```python
from build123d import *

# Parameters (mm, degrees)
F0_R     = 10.7663
F1_DEPTH = 30
F2_DEPTH = 60


# Not quite as in the source:
# - ends of sketch curves that miss each other by under 0.0002 mm in the source are joined


with BuildPart() as f1:
    # F0 (on Front) → F1 (new body)
    with BuildSketch(Plane.XZ):
        with BuildLine():
            ThreePointArc((3.5818546953, 22.2130663561), (17.1295319645, 14.5886645954), (22.5, 0))
            ThreePointArc((22.5, 0), (17.1295319492, -14.5886646134), (3.5818546487, -22.2130663636))
            Line((3.5818546487, -22.2130663636), (45.4461782926, -15.469383066))
            ThreePointArc((45.4461782926, -15.469383066), (29.5242054073, -0.0258695995), (45.3944581798, 15.4707882881))
            Line((45.3944581798, 15.4707882881), (3.5818546953, 22.2130663561))
        make_face()
        with BuildLine():
            ThreePointArc((60.4758162147, 0), (56.0816390892, 10.8026923778), (45.3944581798, 15.4707882881))
            ThreePointArc((45.3944581798, 15.4707882881), (29.5242054073, -0.0258695995), (45.4461782926, -15.469383066))
            ThreePointArc((45.4461782926, -15.469383066), (56.0996815443, -10.7841530557), (60.4758162147, 0))
        make_face()
        with Locations((45, 0)):
            Circle(F0_R, mode=Mode.SUBTRACT)
    extrude(amount=F1_DEPTH)

    # F0 (on Front) → F2 (join)
    with BuildSketch(Plane.XZ):
        with BuildLine():
            ThreePointArc((3.5818546487, -22.2130663636), (17.1295319492, -14.5886646134), (22.5, 0))
            ThreePointArc((22.5, 0), (17.1295319645, 14.5886645954), (3.5818546953, 22.2130663561))
            ThreePointArc((3.5818546953, 22.2130663561), (-22.5, 2.36e-08), (3.5818546487, -22.2130663636))
        make_face()
        with BuildLine():
            ThreePointArc((-9.780757419, 4.5), (0, 10.7663), (9.780757419, 4.5))
            Line((9.780757419, 4.5), (15, 4.5))
            Line((15, 4.5), (15, -4.5))
            Line((15, -4.5), (9.780757419, -4.5))
            ThreePointArc((9.780757419, -4.5), (0, -10.7663), (-9.780757419, -4.5))
            Line((-9.780757419, -4.5), (-15, -4.5))
            Line((-15, -4.5), (-15, 4.5))
            Line((-15, 4.5), (-9.780757419, 4.5))
        make_face(mode=Mode.SUBTRACT)
    extrude(amount=F2_DEPTH)


solid = f1.part
```
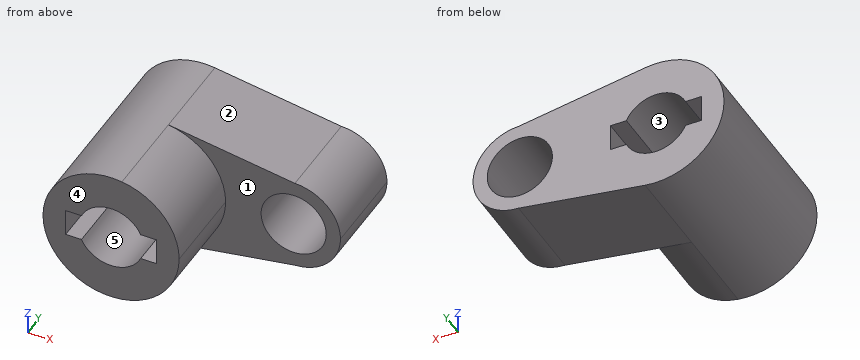
Verification items for the finished model (mm, model axes). Face numbers are marked on the shaded views. A direction names the side the tool comes from. Round coordinates to 2 decimals unless told otherwise and drop trailing zeros. Order: outer loops, then holes, each group sorted by start corner. A loop starts at its lowest first (then second) coordinate and runs counter-clockwise, first axis right, second up. Notation, with made-up numbers: (-8.5, 13) -> (20.5, 13) arc R9 ccw to (20.5, 23) -> close; hole circle Ø3 at (21, 34). An arc over 180 degrees is marked (long way). Put each result on its own line as item: value. Start each with the question number.
(1) Section check C-C (y = -50). Enter the section's corners in (x, z), then the cut area to 3 significant figures.
(2) Material ranges on line 1 along X through (y, z) = (-10, -9); line 2 along Z through (x, y) = (45, -11); line 3 along Y through (x, z) = (17.5, -16), recorded low to high.
(3) Section check B-B (x = 0). Enter the section's corners in (y, z).
(4) Section check A-A (y = -8). Enter the section's corners in (x, z), then the cut area to 3 significant figures.
(5) Draft check along X on the marked faces 1, 2 and 3. Enter one of: +X half, -X half, draft (parallel to the pull), parting line (faces both ways), or undercut.
(6) Section check D-D (z = 8). Enter the section's corners in (x, y), then the cut area to 3 significant figures.
(7) Depth check by flat-ended pin: pin 1 Ø1.5 at (y, z) = (-7, -3.5) entering from -X; pin 2 Ø3 at (y, z) = (-17, 13.5) entering from +X; pin 3 Ø1.6 at (x, y) = (-13.5, -18.5) entering from +Z. Enter the tip coordinate at first touch or a pass-through.
(8) Tool access check on the marked faces 4 and 5. Record the directions out of +Z, -Z, +X, -X, +Y, -Y that give a thin tool (end or side, any length) a straight path to the whole face; none if there is none.
Completed:
1. outline: circle Ø45 at (0, 0); hole (-15, -4.5) -> (-9.78, -4.5) arc R10.77 ccw to (9.78, -4.5) -> (15, -4.5) -> (15, 4.5) -> (9.78, 4.5) arc R10.77 ccw to (-9.78, 4.5) -> (-15, 4.5) -> close
1. area: 1,140 mm2
2. line 1: x = -20.62 to -5.91, 5.91 to 39.09, 50.91 to 57.59
2. line 2: z = -15.54 to -10.77, 10.77 to 15.53
2. line 3: y = -30 to 0
3. outline: (-60, -22.5) -> (0, -22.5) -> (0, -10.77) -> (-60, -10.77) -> close; (-60, 10.77) -> (0, 10.77) -> (0, 22.5) -> (-60, 22.5) -> close
4. outline: (3.58, -22.21) -> (45.45, -15.47) arc R15.48 ccw to (45.39, 15.47) -> (3.58, 22.21) arc R22.5 ccw (long way) to start; hole (-15, -4.5) -> (-9.78, -4.5) arc R10.77 ccw to (9.78, -4.5) -> (15, -4.5) -> (15, 4.5) -> (9.78, 4.5) arc R10.77 ccw to (-9.78, 4.5) -> (-15, 4.5) -> close; hole circle Ø21.53 at (45, 0)
4. area: 2,090 mm2
5. face 1: draft
5. face 2: +X half
5. face 3: undercut
6. outline: (-21.03, -60) -> (-7.21, -60) -> (-7.21, 0) -> (-21.03, 0) -> close; (7.21, -60) -> (21.03, -60) -> (21.03, -30) -> (37.79, -30) -> (37.79, 0) -> (7.21, 0) -> close; (52.21, -30) -> (58.25, -30) -> (58.25, 0) -> (52.21, 0) -> close
6. area: 2,340 mm2
7. pin 1: stops at x = -22.33
7. pin 2: stops at x = 54.77
7. pin 3: stops at z = 18.57
8. face 4: +Z, -Z, +X, -X, -Y
8. face 5: +Y, -Y
